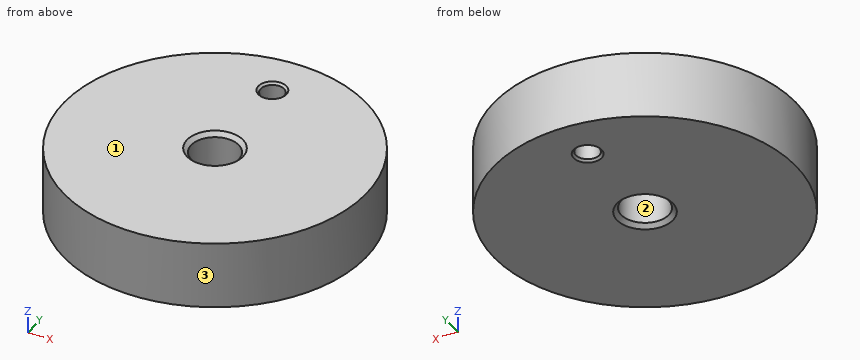
```python
from build123d import *

# Parameters (mm, degrees)
SKETCH1_R           = 27
BOSS_EXTRUDE1_DEPTH = 12


with BuildPart() as part:
    # Sketch1 → Boss-Extrude1 (new body)
    with BuildSketch(Plane.XY):
        Circle(SKETCH1_R)
    extrude(amount=BOSS_EXTRUDE1_DEPTH)

    # Sketch8 → M10 Tapped Hole2 (revolve, cut)
    with BuildSketch(Plane(origin=(0, 0, 12), x_dir=(0, -1, 0), z_dir=(1, 0, 0))):
        Polygon((0, 0), (0, 12), (5, 12), (4.25, 11.25), (4.25, 0.75), (5, 0), align=None)
    revolve(axis=Axis((0, 0, 18.35), (0, 0, -1)), mode=Mode.SUBTRACT)

    # Sketch9 → M5 Tapped Hole1 (revolve, cut)
    with BuildSketch(Plane(origin=(0, 18.69698963, 12), x_dir=(0, -1, 0), z_dir=(1, 0, 0))):
        Polygon((0, 0), (0, 12), (2.5, 12), (2.1, 11.6), (2.1, 0.4), (2.5, 0), align=None)
    revolve(axis=Axis((0, 18.69698963, 18.35), (0, 0, -1)), mode=Mode.SUBTRACT)


solid = part.part
```
Build history of the part. All positions in model axes, mm. Face numbers are marked on the shaded views. Give positions to 0.01 mm unless a question says otherwise; leave off trailing zeros. Loops run counter-clockwise (first coordinate to the right, second up) from the corner with the lowest first, then second, coordinate; pieces in that order, holes last. Notation, with made-up numbers: (22, 43.5) -> (70, 43.5) arc R34 cw to (70, 81.5) -> close; hole circle Ø10 at (76, 49). An arc over 180 degrees is marked (long way). One line per question, with ' | ' between items. Start each with the question number.
1) Cut at D-D (y = -6.5). Give the cut face in (x, z).
2) Cut at C-C (z = 6.25). Give the cut face in (x, y).
3) Probe L1, parallel to Y at x = 0, z = 9; L2, parallel to Y at x = 1, z = 8.25; L3, parallel to X at y = 20.5, z = 2.5. List the from-to ranges inside material, lowest first.
4) Pin check, flat tips, straight feed: pin 1 (1 mm diameter, centred on y = -5, z = 5.5, fed in from +X); pin 2 (2 mm diameter, centred on y = -9.5, z = 6.5, fed in from +X); pin 3 (3.5 mm diameter, centred on x = 0, y = 18.7, fed in from -Z); pin 4 (4 mm diameter, centred on y = 6, z = 2, fed in from +X). Stop position of each tip, or through.
5) Cut at B-B (x = 0). Give the cut face in (y, z), plus the area to 3 significant figures.
6) Two-plate mould, pull along Y, no slides. Class the marked faces 1, 2 and 3: released by +Y, released by -Y, zero draft, split by the parting line, or undercut.
7) Cut at A-A (y = 0). Give the cut face in (x, z).
Return value:
1) outline: (-26.21, 0) -> (26.21, 0) -> (26.21, 12) -> (-26.21, 12) -> close
2) outline: circle Ø54 at (0, 0); hole circle Ø8.5 at (0, 0); hole circle Ø4.2 at (0, 18.7)
3) L1: -27 to -4.25, 4.25 to 16.6, 20.8 to 27 | L2: -26.98 to -4.13, 4.13 to 16.85, 20.54 to 26.98 | L3: -17.57 to -1.08, 1.08 to 17.57
4) pin 1: x = 26.62 | pin 2: x = 25.63 | pin 3: through | pin 4: x = 26.7
5) outline: (-27, 0) -> (-5, 0) -> (-4.25, 0.75) -> (-4.25, 11.25) -> (-5, 12) -> (-27, 12) -> close; (4.25, 0.75) -> (5, 0) -> (16.2, 0) -> (16.6, 0.4) -> (16.6, 11.6) -> (16.2, 12) -> (5, 12) -> (4.25, 11.25) -> close; (20.8, 0.4) -> (21.2, 0) -> (27, 0) -> (27, 12) -> (21.2, 12) -> (20.8, 11.6) -> close | area: 494 mm^2
6) face 1: zero draft | face 2: undercut | face 3: split by the parting line
7) outline: (-27, 0) -> (-5, 0) -> (-4.25, 0.75) -> (-4.25, 11.25) -> (-5, 12) -> (-27, 12) -> close; (4.25, 0.75) -> (5, 0) -> (27, 0) -> (27, 12) -> (5, 12) -> (4.25, 11.25) -> close
